Autodesk Fusion 360 part; units mm, degrees
sketch "Sketch1" plane through (0, 0, 0) normal (0, 1, 0) x (1, 0, 0)
  line L0 (0, 0) -> (20, 0)
  line L1 (20, 0) -> (20, -40)
  line L2 (20, -40) -> (0, -40)
  line L3 (0, -40) -> (0, 0)
  line L4 (20, -40) -> (10, -40)
  line L5 (10, -40) -> (10, 0)
  line L6 (10, -40) -> (10, -30)
  line L7 (10, 0) -> (10, -10)
  circle A0 centre (10, -10) radius 2.75
  circle A1 centre (10, -30) radius 2.75
  circle A2 centre (10, -30) radius 4.75
  circle A3 centre (10, -10) radius 4.75
  dimension "d1" = 20
  dimension "d2" = 40
  dimension "d3" = 10
  dimension "d4" = 10
  dimension "d5" = 10
  dimension "d6" = 5.5
  dimension "d7" = 5.5
  dimension "d10" = 9.5
  dimension "d11" = 9.5
extrude "Extrude1" add sketch "Sketch1" along normal blind 25 contours L0 L2 L3 L5 L6 L7 A2 A3 | L0 L1 L2 L4 L5 L6 L7 A2 A3 | L5 L7 A0 A3 | L5 L7 A0 A3 | L5 L6 A1 A2 | L5 L6 A1 A2
extrude "Extrude2" cut sketch "Sketch1" along normal blind 10 contours L5 L7 A0 A3 | L5 L7 A0 A3 | L5 L6 A1 A2 | L5 L6 A1 A2
sketch "Sketch2" plane through (0, 0, 0) normal (1, 0, 0) x (0, 1, 0)
  line L0 (0, 0) -> (20, 0)
  line L1 (20, 0) -> (20, 40)
  line L2 (20, 40) -> (0, 40)
  line L3 (0, 40) -> (0, 0)
  line L4 (0, 30) -> (10, 30)
  line L5 (0, 10) -> (10, 10)
  circle A0 centre (10, 30) radius 2.35
  circle A1 centre (10, 10) radius 2.35
  dimension "d14" = 20
  dimension "d15" = 10
  dimension "d16" = 10
  dimension "d17" = 4.7
  dimension "d18" = 4.7
sketch "Sketch3" plane through (0, 0, 40) normal (0, 0, 1) x (-1, 0, 0)
  line L0 (0, 0) -> (-20, 0)
  line L1 (-20, 0) -> (-20, -25)
  line L2 (-20, -25) -> (0, -25)
  line L3 (0, -25) -> (0, 0)
  line L4 (-15, 0) -> (-5, 0)
  line L5 (0, -5) -> (0, -15.3305)
  line L6 (-20, -15.3305) -> (-20, -5)
  line L7 (-10.403, -10.0836) -> (-9.4234, -10.0836)
  line L8 (0, -10) -> (0, -15.3305)
  line L9 (-19, -16.3305) -> (-15.6115, -16.3305)
  line L10 (-14.6115, -15.3305) -> (-14.6115, -12.2318)
  line L11 (-1, -16.3305) -> (-4.0034, -16.3305)
  line L12 (-5.0034, -15.3305) -> (-5.0034, -12.4938)
  arc A0 (-5.0034, -12.4938) -> (-14.6115, -12.2318) centre (-9.9132, -16.2396) ccw
  line L13 (-1, -16.3305) -> (-4.0034, -16.3305)
  line L14 (-15.6115, -16.3305) -> (-19, -16.3305)
  line L15 (-1, -16.3305) -> (-4.0034, -16.3305)
  line L16 (-15.6115, -16.3305) -> (-19, -16.3305)
  arc A1 (-15.6115, -16.3305) -> (-14.6115, -15.3305) centre (-15.6115, -15.3305) ccw
  arc A2 (-5.0034, -15.3305) -> (-4.0034, -16.3305) centre (-4.0034, -15.3305) ccw
  arc A3 (-20, -15.3305) -> (-19, -16.3305) centre (-19, -15.3305) ccw
  arc A4 (-1, -16.3305) -> (0, -15.3305) centre (-1, -15.3305) ccw
  arc A5 (-15, 0) -> (-20, -5) centre (-15, -5) ccw
  arc A6 (0, -5) -> (-5, 0) centre (-5, -5) ccw
  dimension "d24" = 1
  dimension "d25" = 1
  dimension "d26" = 5
extrude "Extrude4" add sketch "Sketch3" along normal blind 150 contours L0 L1 L3 L4 L5 L6 L8 L9 L10 L11 L12 A0 L13 L14 L15 L16 A1 A2 A3 A4 A5 A6
sketch "Sketch4" plane through (0, 0, 190) normal (0, 0, 1) x (-1, 0, 0)
  line L0 (0, -15.3305) -> (0, -5)
  arc A0 (0, -5) -> (-5, 0) centre (-5, -5) ccw
  line L1 (-5, 0) -> (-15, 0)
  arc A1 (-15, 0) -> (-20, -5) centre (-15, -5) ccw
  line L2 (-20, -5) -> (-20, -15.3305)
  arc A2 (-20, -15.3305) -> (-19, -16.3305) centre (-19, -15.3305) ccw
  line L3 (-19, -16.3305) -> (-15.6115, -16.3305)
  arc A3 (-15.6115, -16.3305) -> (-14.6115, -15.3305) centre (-15.6115, -15.3305) ccw
  line L4 (-14.6115, -15.3305) -> (-14.6115, -12.2318)
  arc A4 (-5.0034, -12.4938) -> (-14.6115, -12.2318) centre (-9.9132, -16.2396) ccw
  line L5 (-5.0034, -12.4938) -> (-5.0034, -15.3305)
  arc A5 (-5.0034, -15.3305) -> (-4.0034, -16.3305) centre (-4.0034, -15.3305) ccw
  line L6 (-4.0034, -16.3305) -> (-1, -16.3305)
  arc A6 (-1, -16.3305) -> (0, -15.3305) centre (-1, -15.3305) ccw
  circle A7 centre (-9.9132, -16.2396) radius 1.55
  line L7 (0, 0) -> (-63.7918, 0)
  line L8 (-69.7918, -6) -> (-69.7918, -68.86)
  line L9 (-63.7918, -74.86) -> (-6, -74.86)
  line L10 (0, -68.86) -> (0, 0)
  arc A8 (-63.7918, 0) -> (-69.7918, -6) centre (-63.7918, -6) ccw
  arc A9 (-69.7918, -68.86) -> (-63.7918, -74.86) centre (-63.7918, -68.86) ccw
  arc A10 (-6, -74.86) -> (0, -68.86) centre (-6, -68.86) ccw
  arc A11 (0, -5) -> (-5, 0) centre (-5, -5) ccw
  circle A12 centre (-59.9132, -16.2396) radius 1.55
  circle A13 centre (-60, -66.2375) radius 1.55
  circle A14 centre (-9.9132, -66.2396) radius 1.55
  dimension "d29" = 3.1
  dimension "d30" = 50
  dimension "d31" = 50
  dimension "d32" = 6
  dimension "d33" = 3.1
  dimension "d34" = 3.1
  dimension "d35" = 3.1
extrude "Extrude5" add sketch "Sketch4" along normal blind 10 contours L0 A0 L1 A1 L2 A2 L3 A3 L4 A4 L5 A5 L6 A6 L7 L10 A11 | A1 L2 A2 L3 A3 L4 A4 L5 A5 L6 A6 L7 L8 L9 L10 A8 A9 A10
sketch "Sketch5" plane through (0, 0, 0) normal (0, -1, 0) x (1, 0, 0)
  circle A0 centre (10, 30) radius 4.75
  circle A1 centre (10, 10) radius 4.75
  line L0 (20, 0) -> (20, 40)
  line L1 (20, 40) -> (15, 40)
  line L2 (15, 40) -> (15, 190)
  line L3 (15, 190) -> (63.7918, 190)
  line L4 (63.7918, 190) -> (63.7918, 200)
  line L5 (63.7918, 200) -> (5, 200)
  line L6 (5, 200) -> (5, 40)
  line L7 (5, 40) -> (0, 40)
  line L8 (0, 40) -> (0, 0)
  line L9 (0, 0) -> (20, 0)
  line L10 (20, 190) -> (65, 190)
  line L11 (20, 145) -> (20, 190)
  arc A2 (65, 190) -> (20, 145) centre (65, 145) ccw
extrude "Extrude6" add sketch "Sketch5" against normal blind 10 from surface at -5 contours L3 L10 L11 A2
extrude "Extrude7" cut 1 faces at (59.9434, 14.7871, 190) along direction (0, 0, -1) blind 5
Read the model definition and answer for the solid it produces. Units are mm, in the model's axes. A direction names the side the tool comes from. Coordinates: 2 decimals unless noted, no trailing zeros. Write each loop counter-clockwise with the first axis right and the second up, starting at its lowest first coordinate (ties: lowest second). Pieces come first, ordered by that corner, then holes. Notation, with made-up numbers: (-28.5, 81.5) -> (-16.5, 81.5) arc R14 cw to (-16.5, 103.5) -> close; hole circle Ø10 at (66.25, -18.5). An arc over 180 degrees is marked (long way). Return JSON: item names as keys, results as strings.
(1) Each of these flat-tipped pins is pushed along its axis until it touches: P1, Ø6, axis at y = 13.5, z = 77, coming from the +X side; P2, Ø5, axis at x = 59.91, y = 16.24, coming from the -Z side; P3, Ø3.5, axis at x = 9.91, y = 66.24, coming from the -Z side; P4, Ø3.5, axis at x = 10, z = 10, coming from the +Y side. Where does it stop, or does it pass through?
Answers below:
{"P1": "x = 20", "P2": "z = 189.41", "P3": "z = 190", "P4": "through"}
(2) The part is cut by section B-B on z = 77.5. Give the vertices of the cut face in (x, y).
Answers below:
{"outline": "(0, 5) arc R5 ccw to (5, 0) -> (15, 0) arc R5 ccw to (20, 5) -> (20, 15.33) arc R1 ccw to (19, 16.33) -> (15.61, 16.33) arc R1 ccw to (14.61, 15.33) -> (14.61, 12.23) arc R6.18 cw to (5, 12.49) -> (5, 15.33) arc R1 ccw to (4, 16.33) -> (1, 16.33) arc R1 ccw to (0, 15.33) -> close"}
(3) The part is cut by section A-A on z = 10. Give the vertices of the cut face in (x, y), then the cut area to 4 significant figures.
Answers below:
{"outline": "(0, 0) -> (5.25, 0) -> (5.25, 10) -> (7.25, 10) -> (7.25, 25) -> (0, 25) -> close; (12.75, 10) -> (14.75, 10) -> (14.75, 0) -> (20, 0) -> (20, 25) -> (12.75, 25) -> close", "area": "322.5 mm^2"}
(4) The part is cut by section D-D on x = 44. Give the vertices of the cut face in (y, z), then the cut area to 3 significant figures.
Answers below:
{"outline": "(0, 190) -> (5, 190) -> (5, 184.8) -> (15, 184.8) -> (15, 190) -> (74.86, 190) -> (74.86, 200) -> (0, 200) -> close", "area": "801 mm^2"}
(5) The part is cut by section C-C on y = 34.5. Give the vertices of the cut face in (x, z).
Answers below:
{"outline": "(0, 190) -> (69.79, 190) -> (69.79, 200) -> (0, 200) -> close"}
(6) For a pull along X with two mould halves and no side action, classify faces 6 (the flat face through (29, 15, 179)), 7 (the cylindrical face through (11.48, 17.4, 12.32)), 8 (the cylindrical face through (33.532, 9.93, 177.168)) as pulls with the +X half, pulls with the -X half, needs draft (parallel to the pull), parting line crosses it, or undercut.
Answers below:
{"face 6": "needs draft", "face 7": "undercut", "face 8": "pulls with the +X half"}
(7) Consider line 1 along Z through (x, y) = (10, 3.5); line 2 along Z through (x, y) = (40, 33); line 3 along X through (y, z) = (8, 54). Determine where each line is inside the solid, lowest interval first. Write a range as from..to.
Answers below:
{"line 1": "0..5.25, 14.75..25.25, 34.75..200", "line 2": "190..200", "line 3": "0..20"}
(8) Which of the six approach directions +Z, -Z, +X, -X, +Y, -Y give full straight-line access (tool end or side, diameter ignored) to faces 1 (the flat face through (29, 5, 179)), 2 (the cylindrical face through (2, 1, 119)), 3 (the flat face through (10, 10, 33)), 4 (the flat face through (17, 16.33, 114)), 5 (the cylindrical face through (9.822, 10.065, 113.95))?
Answers below:
{"face 1": "-Z, +X, -Y", "face 2": "+Z, -X, -Y", "face 3": "-Y", "face 4": "+X, -X, +Y", "face 5": "+Y"}
